Could you check a few things on this model? Use its own coordinates, in mm. A direction names the side the tool comes from. Round coordinates to 2 decimals unless told otherwise and drop trailing zeros. Loops run counter-clockwise (first coordinate to the right, second up) from the corner with the lowest first, then second, coordinate; pieces in that order, holes last. Notation, with made-up numbers: (-26.5, 23) -> (-8.5, 23) arc R27 ccw to (-8.5, 42) -> close; hole circle Ø11 at (45.25, -21.5). An arc over 180 degrees is marked (long way). Put each result on its own line as item: value. Start each with the question number.
1. Imagine slicing it at C-C, the plane y = 21. Please give me the cut outline in (x, z), and give its area (3 significant figures).
2. I need wall thicknesses on line 1 (Z direction, x = 9.5, y = 16); line 2 (X direction, y = 0, z = 9.5); line 3 (X direction, y = 0, z = 9). Which ranges of each line are inside material? Lowest first, please. Write a range as [from, to].
3. Imagine slicing it at D-D, the plane z = 11. Please give me the cut outline in (x, y).
4. Which directions (+Z, -Z, +X, -X, +Y, -Y) give clear straight access to the entire face, cutting with the end or side of a thin tool? Please do faces 1 (the flat face through (10.2, -6.26, 10.12)), 2 (the flat face through (0, 0, 6.35)), 3 (the flat face through (-12.7, -6, 7)).
5. I'm going to push flat-ended pins straight in: P1, Ø11.5, axis at x = 0, y = 0, coming from the -Z side; P2, Ø1, axis at x = 13.5, z = 3.5, coming from the +Y side; P3, Ø4, axis at x = 14, y = 3.5, coming from the +Z side; P4, Ø1.5, axis at x = -6, z = 5, coming from the +Y side. Where does each tip first touch, or does it pass through?
6. Imagine slicing it at B-B, the plane z = 4.5. Please give me the cut outline in (x, y), and give its area (3 significant figures).
7. If we mould it in two halves opening along Y, with no side actions, what happens to faces 4 (the flat face through (5.402, 18.522, 6.403)), 5 (the flat face through (-5.6, -17.54, 10.2)), 6 (the cylindrical face through (-0.661, 5.037, 9.481))? For each: pulls with the +Y half, pulls with the -Y half, needs draft (parallel to the pull), parting line crosses it, or undercut.
8. Imagine slicing it at A-A, the plane z = 8.5. Please give me the cut outline in (x, y), and give its area (3 significant figures).
```python
from build123d import *

# Parameters (mm, degrees)
F0_W         = 25.4
F0_H         = 50.8
F0_R         = 5.08
F1_DEPTH     = 12.7
F3_DEPTH     = 25.4
F4_T1_DEPTH  = 47.9732038629
F4_T3_DEPTH  = 31.5130991577
F4_T5_DEPTH  = 42.2974691352
F4_T7_DEPTH  = 42.2974691352
F4_T9_DEPTH  = 62.5709452641
F4_T11_DEPTH = 62.5736078482
F4_T16_DEPTH = 31.520364883
F4_T21_DEPTH = 31.520364883
F5_R         = 19.9015863144
F6_DEPTH     = 6.35
F7_R         = 1.27


# Not quite as in the source:
# - a fillet or chamfer that OpenCascade refuses, or shapes differently, is made with other operations: its cross-section is extruded or revolved along the edge and cut away or added


with BuildPart() as f1:
    # F0 (on Top) → F1 (new body)
    with BuildSketch(Plane.XY):
        Rectangle(F0_W, F0_H)
        Circle(F0_R, mode=Mode.SUBTRACT)
    extrude(amount=F1_DEPTH)

    # F2 (on face) → F3 (cut)
    with BuildSketch(Plane.XY.offset(12.7)):
        Polygon((-12.7, 25.4), (-12.7, 0), (-2.6996657252, 25.4), align=None)
        Polygon((-2.6924, -25.4), (-12.7, -12.7), (-12.7, -25.4), align=None)
        Polygon((12.7, -12.7), (2.6924, -25.4), (12.7, -25.4), align=None)
        Polygon((12.7, 25.4), (2.6924, 25.4), (12.7, 0), align=None)
    extrude(amount=-F3_DEPTH, mode=Mode.SUBTRACT)

    # F4: chamfer of 5.08 on 8 edges, made by hand

    # F4_s2 → F4_t1 (cut)
    with BuildSketch(Plane.XZ.offset(-22.2090542841)):
        Polygon((-7.62, 12.7), (-12.7, 7.62), (-12.7, 12.7), align=None)
        Polygon((12.7, 7.62), (7.62, 12.7), (12.7, 12.7), align=None)
    extrude(amount=F4_T1_DEPTH, mode=Mode.SUBTRACT)

    # F4_s4 → F4_t3 (cut)
    with BuildSketch(Plane.YZ.offset(-15.7565495789)):
        Polygon((-20.32, 12.7), (-25.4, 7.62), (-25.4, 12.7), align=None)
    extrude(amount=F4_T3_DEPTH, mode=Mode.SUBTRACT)

    # F4_s6 → F4_t5 (cut)
    with BuildSketch(Plane(origin=(6.7769328826, 8.6001686327, 0), x_dir=(0, 0, 1), z_dir=(-0.6189309664, -0.7854453888, 0))):
        Polygon((12.7, -12.7555797114), (7.62, -17.8355797114), (12.7, -17.8355797114), align=None)
    extrude(amount=F4_T5_DEPTH, mode=Mode.SUBTRACT)

    # F4_s8 → F4_t7 (cut)
    with BuildSketch(Plane(origin=(19.4022805654, -24.6221834587, 0), x_dir=(0, 0, 1), z_dir=(-0.6189309664, 0.7854453888, 0))):
        Polygon((12.7, -12.7555797114), (7.62, -17.8355797114), (12.7, -17.8355797114), align=None)
    extrude(amount=F4_T7_DEPTH, mode=Mode.SUBTRACT)

    # F4_s10 → F4_t9 (cut)
    with BuildSketch(Plane(origin=(-9.8405603892, -24.994187896, 0), x_dir=(0, 0, 1), z_dir=(0.3663429193, 0.9304799114, 0))):
        Polygon((12.7, -6.7370948746), (7.62, -11.8170948746), (12.7, -11.8170948746), align=None)
    extrude(amount=F4_T9_DEPTH, mode=Mode.SUBTRACT)

    # F4_s12 → F4_t11 (cut)
    with BuildSketch(Plane(origin=(-13.0899935353, 33.2233338458, 0), x_dir=(0, 0, 1), z_dir=(0.36657333, -0.9303891625, 0))):
        Polygon((7.62, -11.8159423639), (12.7, -6.7359423639), (12.7, -11.8159423639), align=None)
    extrude(amount=F4_T11_DEPTH, mode=Mode.SUBTRACT)


with BuildPart() as f4_tool14:
    # F4_s15 → F4_t16 (new body)
    with BuildSketch(Plane.YZ.offset(15.7565495789)):
        Polygon((20.32, 12.7), (25.4, 7.62), (25.4, 12.7), align=None)
    extrude(amount=-F4_T16_DEPTH)

    split(bisect_by=Plane(origin=(9.0414950692, 3.5623490573, 9.7179711819), x_dir=(-0.36657333, 0.9303891625, 0), z_dir=(0.657884486, 0.2592064875, 0.7071067812)), keep=Keep.TOP)


with BuildPart() as f1_1:
    add(f1.part)

    # F4_t13: cut F4_tool14
    add(f4_tool14.part, mode=Mode.SUBTRACT)


with BuildPart() as f4_tool19:
    # F4_s20 → F4_t21 (new body)
    with BuildSketch(Plane.YZ.offset(15.7565495789)):
        Polygon((20.32, 12.7), (25.4, 7.62), (25.4, 12.7), align=None)
    extrude(amount=-F4_T21_DEPTH)

    split(bisect_by=Plane(origin=(-9.0429131582, 3.5603210394, 9.7185474373), x_dir=(-0.3663429193, -0.9304799114, 0), z_dir=(-0.6579486551, 0.2590435625, 0.7071067812)), keep=Keep.TOP)


with BuildPart() as f1_2:
    add(f1_1.part)

    # F4_t18: cut F4_tool19
    add(f4_tool19.part, mode=Mode.SUBTRACT)

    # F5 (on Top) → F6 (join)
    with BuildSketch(Plane.XY):
        Circle(F5_R)
    extrude(amount=F6_DEPTH)

    # F7
    f7_edges = [f1_2.edges().sort_by_distance(p)[0] for p in [
        (19.817994, 1.822158, 0),
        (19.817994, 1.822158, 6.35),
        (-19.818285, 1.818991, 6.35),
        (-19.818285, 1.818991, 0),
    ]]
    fillet(f7_edges, radius=F7_R)


solid = f1_2.part
```
Entries:
1. outline: (-4.43, 0) -> (4.43, 0) -> (4.43, 7.62) -> (0, 11.74) -> (-4.43, 7.62) -> close
1. area: 85.7 mm^2
2. line 1: [0, 6.35]
2. line 2: [-10.68, -5.08], [5.08, 10.68]
2. line 3: [-11.22, -5.08], [5.08, 11.22]
3. outline: (-9.32, -11.53) -> (-1.05, -22.02) -> (1.05, -22.02) -> (9.32, -11.53) -> (9.32, -0.64) -> (0, 23.02) -> (-9.32, -0.64) -> close; hole circle Ø10.16 at (0, 0)
4. face 1: +Z, +X, +Y, -Y
4. face 2: +Z
4. face 3: +Z, -X, +Y, -Y
5. P1: z = 0
5. P2: y = 15.07
5. P3: z = 6.35
5. P4: y = 19.2
6. outline: (-8.54, -17.97) -> (-2.69, -25.4) -> (2.69, -25.4) -> (8.54, -17.97) arc R19.9 ccw to (5.12, 19.23) -> (2.69, 25.4) -> (-2.7, 25.4) -> (-5.13, 19.23) arc R19.9 ccw to start
6. area: 1,350 mm^2
7. face 4: pulls with the +Y half
7. face 5: pulls with the -Y half
7. face 6: undercut
8. outline: (-11.82, -12.39) -> (-2.27, -24.52) -> (2.27, -24.52) -> (11.82, -12.39) -> (11.82, -0.17) -> (1.75, 25.4) -> (-1.75, 25.4) -> (-11.82, -0.17) -> close; hole circle Ø10.16 at (0, 0)
8. area: 726 mm^2
